The listing builds one solid part. Answer for the finished solid, in the listing's coordinates (mm). Face numbers are marked on the shaded views. A direction names the side the tool comes from. Round coordinates to 2 decimals unless told otherwise and drop trailing zeros. Loops run counter-clockwise (first coordinate to the right, second up) from the corner with the lowest first, then second, coordinate; pieces in that order, holes last. Notation, with made-up numbers: (-14.75, 58) -> (-8.75, 58) arc R17 cw to (-8.75, 77) -> close; hole circle Ø6 at (-16, -24). An arc over 180 degrees is marked (long way). Use a Markdown table: item, result. Add a question column.
Q1. Section D-D on x = -1.25 is taken. Give the vertices of the cut face in (y, z).
Q2. Which of the six approach directions +Z, -Z, +X, -X, +Y, -Y give full straight-line access (tool end or side, diameter ignored) to the marked faces 1 and 2?
Q3. For a pull along Z with two mould halves and no side action, classify the marked faces 3, 4, 5 and 6 as released by +Z, released by -Z, zero draft, split by the parting line, or undercut.
Q4. Given pin 1 Ø1.5 at (y, z) = (0.5, 1) entering from -X, flat-ended and moving along its own axis, determine where the tip first touches the part or whether it passes through.
Q5. Section A-A on x = 0 is taken. Give the vertices of the cut face in (y, z), then the cut area to 3 significant figures.
Q6. Section B-B on y = 0.4 is taken. Give the vertices of the cut face in (x, z).
Q7. Section C-C on z = 1.95 is taken. Give the vertices of the cut face in (x, y).
Q8. Consider line 1 (Y direction, x = -1.75, z = 2.2); line 2 (X direction, y = 2.35, z = 0.5); line 3 (Z direction, x = 1, y = 3.85). Determine where each line is inside the solid, lowest interval first.
from build123d import *

# Parameters (mm, degrees)
BOSS_EXTRU_1_DEPTH      = 3
BOSS_EXTRU_2_START      = 3
ESQUISSE2_R             = 2.6
ESQUISSE2_R_2           = 1.5
BOSS_EXTRU_2_DEPTH      = 1
ESQUISSE3_R             = 1.5
ENL_V_MAT_EXTRU_1_DEPTH = 6.800502852


with BuildPart() as part:
    # Esquisse1 → Boss.-Extru.1 (new body)
    with BuildSketch(Plane(origin=(0, 0, 0), x_dir=(1, 0, 0), z_dir=(0, 1, 0))):
        Polygon((3.175426481, 0), (1.58771324, 2.75), (-1.58771324, 2.75), (-3.175426481, 0), (-1.58771324, -2.75), (1.58771324, -2.75), align=None)
    extrude(amount=BOSS_EXTRU_1_DEPTH)

    # Esquisse2 → Boss.-Extru.2 (add)
    with BuildSketch(Plane(origin=(0, 0, 0), x_dir=(1, 0, 0), z_dir=(0, 1, 0)).offset(BOSS_EXTRU_2_START)):
        with Locations(Location((0, 0, 0), (0, 0, 270))):
            Circle(ESQUISSE2_R)
        with Locations(Location((0, 0, 0), (0, 0, 270))):
            Circle(ESQUISSE2_R_2, mode=Mode.SUBTRACT)
    extrude(amount=BOSS_EXTRU_2_DEPTH)

    # Esquisse3 → Enlèv. mat.-Extru.1 (cut, through all)
    with BuildSketch(Plane(origin=(0, 0, 0), x_dir=(1, 0, 0), z_dir=(0, 1, 0))):
        with Locations(Location((0, 0, 0), (0, 0, 270))):
            Circle(ESQUISSE3_R)
    extrude(amount=ENL_V_MAT_EXTRU_1_DEPTH, mode=Mode.SUBTRACT)


solid = part.part
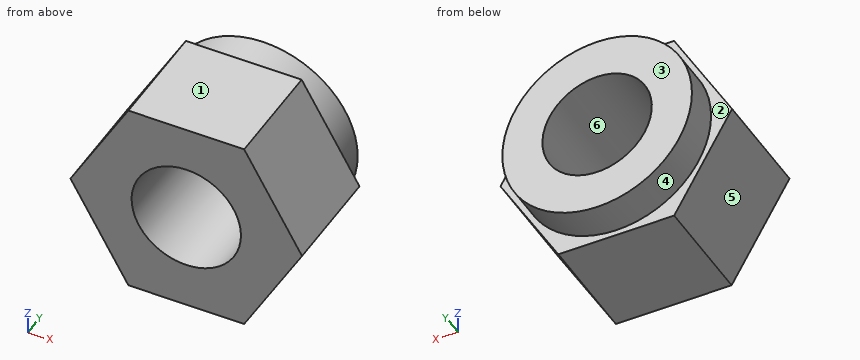
Checked values:
| question | item | result |
|---|---|---|
| 1 | outline | (0, -2.75) -> (3, -2.75) -> (3, -2.28) -> (4, -2.28) -> (4, -0.83) -> (0, -0.83) -> close; (0, 0.83) -> (4, 0.83) -> (4, 2.28) -> (3, 2.28) -> (3, 2.75) -> (0, 2.75) -> close |
| 2 | face 1 | +Z, +X, -X, +Y, -Y |
| 2 | face 2 | +Y |
| 3 | face 3 | zero draft |
| 3 | face 4 | split by the parting line |
| 3 | face 5 | released by -Z |
| 3 | face 6 | undercut |
| 4 | pin 1 | stops at x = -3.03 |
| 5 | outline | (0, -2.75) -> (3, -2.75) -> (3, -2.6) -> (4, -2.6) -> (4, -1.5) -> (0, -1.5) -> close; (0, 1.5) -> (4, 1.5) -> (4, 2.6) -> (3, 2.6) -> (3, 2.75) -> (0, 2.75) -> close |
| 5 | area | 9.70 mm2 |
| 6 | outline | (-3.18, 0) -> (-1.59, -2.75) -> (1.59, -2.75) -> (3.18, 0) -> (1.59, 2.75) -> (-1.59, 2.75) -> close; hole circle Ø3 at (0, 0) |
| 7 | outline | (-2.05, 0) -> (2.05, 0) -> (2.05, 3) -> (1.72, 3) -> (1.72, 4) -> (-1.72, 4) -> (-1.72, 3) -> (-2.05, 3) -> close |
| 8 | line 1 | y = 0 to 3 |
| 8 | line 2 | x = -2.89 to -1.41, 1.41 to 2.89 |
| 8 | line 3 | z = -2.4 to -1.12, 1.12 to 2.4 |
